Could you check a few things on this model? Use its own coordinates, in mm. Round coordinates to 2 decimals unless told otherwise and drop trailing zeros. Write each loop counter-clockwise with the first axis right and the second up, starting at its lowest first coordinate (ties: lowest second). Pieces come first, ordered by that corner, then holes. Notation, with made-up numbers: (47.25, -28.5) - (57.25, -28.5) arc R36 ccw to (57.25, 5.5) - close; hole circle Ø10 at (19.5, -38). An arc over 180 degrees is marked (long way). Write each question's results on one line, items separated by ' | '. Start each with the question number.
(1) For P1, Ø1, axis at x = 2, z = -42.5, coming from the -Y side; P2, Ø1, axis at x = 5, y = 4, coming from the +Z side; P3, Ø2.5, axis at y = -0.5, z = -59, coming from the +X side (3 decimals), each with a flat end and sliding along its axis, tell me the tip position at first contact or that it passes through.
(2) Imagine slicing it at B-B on z = -25.5. Write out the boundary of the cut face in (x, y), then the cut area to 3 significant figures.
(3) Imagine slicing it at A-A on y = 0. Write out the boundary of the cut face in (x, z) (3 decimals).
(4) Please list where these lines run through material, in increasing order: line 1 (Y direction, x = 2.5, z = -27); line 2 (Y direction, x = 0.25, z = -17); line 3 (X direction, y = 4.75, z = -22). Write a range as [from, to].
```python
from build123d import *

# Parameters (mm, degrees)
SKETCH_1_W          = 67.75
SKETCH_1_H          = 6.35
CHAMFER_1_SIZE      = 0.5
CUT_EXTRUDE_1_DEPTH = 1.075


with BuildPart() as part:
    # Эскиз1 → Повернуть1 (revolve)
    with BuildSketch(Plane(origin=(0, 0, 0), x_dir=(0, 0, -1), z_dir=(1, 0, 0)), mode=Mode.PRIVATE) as revolve_1_sk:
        with Locations((33.875, 3.175)):
            Rectangle(SKETCH_1_W, SKETCH_1_H)
    revolve(revolve_1_sk.sketch.rotate(Axis((0, 0, 0), (0, 0, -1)), 90), axis=Axis((0, 0, 0), (0, 0, -1)))

    # Фаска1
    chamfer_1_edges = [part.edges().sort_by_distance(p)[0] for p in [
        (-6.35, 0, 0),
        (-6.35, 0, -67.75),
    ]]
    chamfer(chamfer_1_edges, length=CHAMFER_1_SIZE)

    # Эскиз2 → Вырез-Вытянуть1 (cut)
    with BuildSketch(Plane(origin=(6.35, 0, 0), x_dir=(0, 0, -1), z_dir=(1, 0, 0))):
        with BuildLine():
            Line((53.75, 2.5), (60.75, 2.5))
            ThreePointArc((60.75, 2.5), (63.25, 0), (60.75, -2.5))
            Line((60.75, -2.5), (53.75, -2.5))
            ThreePointArc((53.75, -2.5), (51.25, 0), (53.75, 2.5))
        make_face()
    extrude(amount=-CUT_EXTRUDE_1_DEPTH, mode=Mode.SUBTRACT)


solid = part.part
```
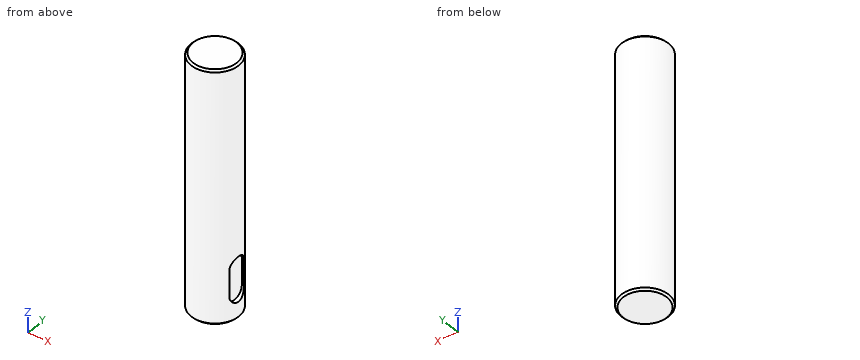
Response:
1) P1: y = -6.17 | P2: z = -0.05 | P3: x = 5.275
2) outline: circle Ø12.7 at (0, 0) | area: 127 mm²
3) outline: (-6.35, -67.25) - (-5.85, -67.75) - (5.85, -67.75) - (6.35, -67.25) - (6.35, -63.25) - (5.275, -63.25) - (5.275, -51.25) - (6.35, -51.25) - (6.35, -0.5) - (5.85, 0) - (-5.85, 0) - (-6.35, -0.5) - close
4) line 1: [-5.84, 5.84] | line 2: [-6.35, 6.35] | line 3: [-4.21, 4.21]
